The listing builds one solid part. Answer for the finished solid, in the listing's coordinates (mm). Face numbers are marked on the shaded views. A direction names the side the tool comes from. Coordinates: 2 decimals unless noted, no trailing zeros. Loops run counter-clockwise (first coordinate to the right, second up) from the corner with the lowest first, then second, coordinate; pieces in that order, holes last. Notation, with made-up numbers: (-3, 55) - (5, 55) arc R21 ccw to (5, 66) - close; hole circle Ø9 at (6, 81). An arc over 180 degrees is marked (long way). Put each result on its own line as item: value.
```python
from build123d import *

# Parameters (mm, degrees)
SKETCH1_W                       = 40
SKETCH1_H                       = 50
SKETCH1_R                       = 45
BOSS_EXTRUDE1_DEPTH             = 50
SKETCH3_R                       = 13
CUT_EXTRUDE1_DEPTH              = 130
BOSS_EXTRUDE3_DEPTH             = 42
BOSS_EXTRUDE3_DEPTH_BACK        = 10
SKETCH6_W                       = 7
SKETCH6_H                       = 4
SKETCH6_H_2                     = 10
SKETCH6_W_2                     = 3
CUT_EXTRUDE2_DEPTH              = 11
CUT_EXTRUDE2_DEPTH_BACK         = 43
SKETCH5_W                       = 42
SKETCH5_H                       = 40
SKETCH9_R                       = 1.5
CUT_EXTRUDE4_DEPTH              = 10
SKIZZE1_R                       = 6
SCHNITT_LINEAR_AUSTRAGEN1_DEPTH = 50
AUFSATZ_LINEAR_START            = 36
SKIZZE2_R                       = 17.5
SKIZZE2_R_2                     = 6
AUFSATZ_LINEAR_AUSTRAGEN1_DEPTH = 36
AUFSATZ_LINEAR_START_2          = 1
SKIZZE3_R                       = 21.5
SKIZZE3_R_2                     = 17.5
AUFSATZ_LINEAR_AUSTRAGEN2_DEPTH = 1
SKIZZE4_R                       = 1.65
SCHNITT_LINEAR_AUSTRAGEN2_DEPTH = 15
SKIZZE5_R                       = 18.5
SCHNITT_LINEAR_AUSTRAGEN3_DEPTH = 7
SKIZZE6_R                       = 17.25
SCHNITT_LINEAR_AUSTRAGEN4_DEPTH = 1


with BuildPart() as part:
    # Sketch1 → Boss-Extrude1 (new body)
    with BuildSketch(Plane.XY):
        with Locations((70, 60)):
            Rectangle(SKETCH1_W, SKETCH1_H)
        with BuildLine():
            Line((44.614473451, -5.877819215), (50, 35))
            Line((50, 35), (50, 85))
            Line((50, 85), (10, 85))
            Line((10, 85), (-35.25108577, 27.970715973))
            ThreePointArc((-35.25108577, 27.970715973), (14.810488519, 42.492933881), (45, 0))
            ThreePointArc((45, 0), (44.903514925, -2.945224501), (44.614473451, -5.877819215))
        make_face()
        Circle(SKETCH1_R)
    extrude(amount=BOSS_EXTRUDE1_DEPTH)

    # Sketch3 → Cut-Extrude1 (cut)
    with BuildSketch(Plane(origin=(90, 0, 0), x_dir=(0, 0, -1), z_dir=(1, 0, 0))):
        with Locations(Location((-25, 60, 0), (0, 0, 90))):
            Circle(SKETCH3_R)
    extrude(amount=-CUT_EXTRUDE1_DEPTH, mode=Mode.SUBTRACT)

    # Sketch6 → Boss-Extrude3 (add, two sides: drawn at the far end of the back side and taken through both)
    with BuildSketch(Plane(origin=(0, 85, 0), x_dir=(1, 0, 0), z_dir=(0, 1, 0)).offset(-BOSS_EXTRUDE3_DEPTH_BACK)):
        Polygon((43, -4), (43, 0), (10, 0), (10, -4), (13, -4), align=None)
        with Locations((6.5, -2)):
            Rectangle(SKETCH6_W, SKETCH6_H)
        with Locations((6.5, -9)):
            Rectangle(SKETCH6_W, SKETCH6_H_2)
        with Locations((11.5, -9)):
            Rectangle(SKETCH6_W_2, SKETCH6_H_2)
        with Locations((11.5, -41)):
            Rectangle(SKETCH6_W_2, SKETCH6_H_2)
        with Locations((6.5, -41)):
            Rectangle(SKETCH6_W, SKETCH6_H_2)
        with Locations((6.5, -48)):
            Rectangle(SKETCH6_W, SKETCH6_H)
        Polygon((13, -46), (10, -46), (10, -50), (43, -50), (43, -46), align=None)
    extrude(amount=BOSS_EXTRUDE3_DEPTH + BOSS_EXTRUDE3_DEPTH_BACK)

    # Sketch5 → Cut-Extrude2 (cut, two sides: drawn at the far end of the back side and taken through both)
    with BuildSketch(Plane.ZY.offset(40).offset(-CUT_EXTRUDE2_DEPTH_BACK)):
        with Locations((25, 60)):
            Rectangle(SKETCH5_W, SKETCH5_H)
    extrude(amount=CUT_EXTRUDE2_DEPTH + CUT_EXTRUDE2_DEPTH_BACK, mode=Mode.SUBTRACT)

    # Sketch9 → Cut-Extrude4 (cut)
    with BuildSketch(Plane(origin=(13, 0, 0), x_dir=(0, 0, -1), z_dir=(1, 0, 0))):
        with Locations(Location((-9.500219356, 121.499780644, 0), (0, 0, 90))):
            Circle(SKETCH9_R)
        with Locations(Location((-9.500219356, 90.500219356, 0), (0, 0, 90))):
            Circle(SKETCH9_R)
        with Locations(Location((-40.499780644, 90.500219356, 0), (0, 0, 90))):
            Circle(SKETCH9_R)
        with Locations(Location((-40.499780644, 121.499780644, 0), (0, 0, 90))):
            Circle(SKETCH9_R)
    extrude(amount=-CUT_EXTRUDE4_DEPTH, mode=Mode.SUBTRACT)

    # Skizze1 → Schnitt-Linear austragen1 (cut)
    with BuildSketch(Plane(origin=(0, 0, 0), x_dir=(-1, 0, 0), z_dir=(0, 0, -1))):
        Circle(SKIZZE1_R)
    extrude(amount=-SCHNITT_LINEAR_AUSTRAGEN1_DEPTH, mode=Mode.SUBTRACT)

    # Skizze2 → Aufsatz-Linear austragen1 (add)
    with BuildSketch(Plane(origin=(0, 0, 0), x_dir=(-1, 0, 0), z_dir=(0, 0, -1)).offset(AUFSATZ_LINEAR_START)):
        with Locations(Location((0, 0, 0), (0, 0, 180))):
            Circle(SKIZZE2_R)
        Circle(SKIZZE2_R_2, mode=Mode.SUBTRACT)
    extrude(amount=-AUFSATZ_LINEAR_AUSTRAGEN1_DEPTH)

    # Skizze3 → Aufsatz-Linear austragen2 (add)
    with BuildSketch(Plane(origin=(0, 0, 0), x_dir=(-1, 0, 0), z_dir=(0, 0, -1)).offset(AUFSATZ_LINEAR_START_2)):
        with Locations(Location((0, 0, 0), (0, 0, 180))):
            Circle(SKIZZE3_R)
        Circle(SKIZZE3_R_2, mode=Mode.SUBTRACT)
    extrude(amount=-AUFSATZ_LINEAR_AUSTRAGEN2_DEPTH)

    # Skizze4 → Schnitt-Linear austragen2 (cut)
    with BuildSketch(Plane(origin=(0, 0, -36), x_dir=(-1, 0, 0), z_dir=(0, 0, -1))):
        with Locations((-11.75, 0)):
            Circle(SKIZZE4_R)
        with Locations((-5.875, 10.175798494)):
            Circle(SKIZZE4_R)
        with Locations((5.875, 10.175798494)):
            Circle(SKIZZE4_R)
        with Locations((11.75, 0)):
            Circle(SKIZZE4_R)
        with Locations((5.875, -10.175798494)):
            Circle(SKIZZE4_R)
        with Locations((-5.875, -10.175798494)):
            Circle(SKIZZE4_R)
    extrude(amount=-SCHNITT_LINEAR_AUSTRAGEN2_DEPTH, mode=Mode.SUBTRACT)

    # Skizze5 → Schnitt-Linear austragen3 (cut)
    with BuildSketch(Plane(origin=(90, 0, 0), x_dir=(0, 0, -1), z_dir=(1, 0, 0))):
        with Locations(Location((-25, 60, 0), (0, 0, 90))):
            Circle(SKIZZE5_R)
    schnitt_linear_austragen3 = extrude(amount=-SCHNITT_LINEAR_AUSTRAGEN3_DEPTH, mode=Mode.SUBTRACT)

    # Skizze6 → Schnitt-Linear austragen4 (cut)
    with BuildSketch(Plane(origin=(83, 0, 0), x_dir=(0, 0, -1), z_dir=(1, 0, 0))):
        with Locations(Location((-25, 60, 0), (0, 0, 90))):
            Circle(SKIZZE6_R)
    schnitt_linear_austragen4 = extrude(amount=-SCHNITT_LINEAR_AUSTRAGEN4_DEPTH, mode=Mode.SUBTRACT)

    # Spiegeln1: Schnitt-Linear austragen3, Schnitt-Linear austragen4 across plane
    add(schnitt_linear_austragen3.mirror(Plane(origin=(46.5, 0, 0), x_dir=(0, 0, 1), z_dir=(1, 0, 0))), mode=Mode.SUBTRACT)
    add(schnitt_linear_austragen4.mirror(Plane(origin=(46.5, 0, 0), x_dir=(0, 0, 1), z_dir=(1, 0, 0))), mode=Mode.SUBTRACT)


solid = part.part
```
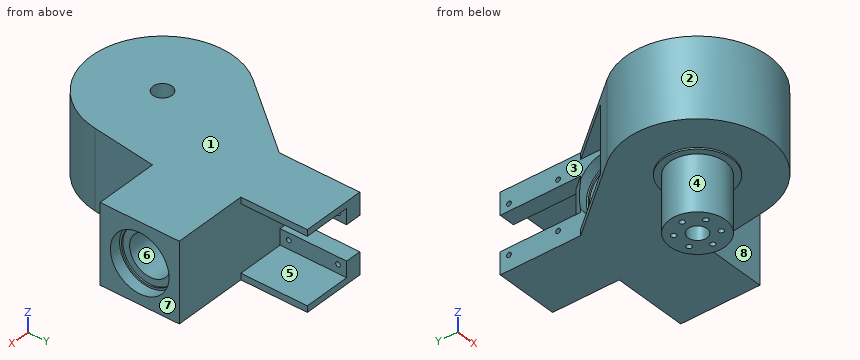
1) For the marked faces 4, 5, 6, 7 and 8, determine the directions among +Z, -Z, +X, -X, +Y, -Y from which every point of the face is accessible in a straight line to the end or side of a thin tool.
Found:
face 4: -Z
face 5: +X, +Y
face 6: +X, -X
face 7: +Z, -Z, +X, +Y, -Y
face 8: +Z, -Z, +X, -Y
2) The part is cut by section D-D (x = 38). Give the vertices of the cut face in (y, z).
Found:
outline: (-24.1, 0) - (127, 0) - (127, 4) - (85, 4) - (85, 46) - (127, 46) - (127, 50) - (-24.1, 50) - close; hole circle Ø26 at (60, 25)
3) Straight lines are drawn through the part: L1, parallel to Z at x = 39, y = 60; L2, parallel to Z at x = -29, y = 18; L3, parallel to X at y = 72, z = 6. For each, find the intervals that lie inside material, in ascending order. Write a range as [from, to].
Found:
L1: z = [0, 12], [38, 50]
L2: z = [0, 50]
L3: x = [3, 90]
4) Each of these flat-tipped pins is pushed along its axis until it touches: pin 1 (17 mm diameter, centred on y = 56.5, z = 29, fed in from +X); pin 2 (10.5 mm diameter, centred on y = 52.5, z = 33.5, fed in from -X); pin 3 (12 mm diameter, centred on x = 61, z = 25, fed in from -Y); pin 4 (1.5 mm diameter, centred on x = 3, y = -3.5, fed in from +Z). Where does it stop, or does it pass through?
Found:
pin 1: stops at x = 82
pin 2: stops at x = 11
pin 3: stops at y = 35
pin 4: passes through
5) The part is cut by section C-C (x = 0). Give the vertices of the cut face in (y, z).
Found:
outline: (-45, 0) - (-21.5, 0) - (-21.5, -1) - (-17.5, -1) - (-17.5, -36) - (-6, -36) - (-6, 50) - (-45, 50) - close; (6, -36) - (17.5, -36) - (17.5, -1) - (21.5, -1) - (21.5, 0) - (72.4, 0) - (72.4, 4) - (40, 4) - (40, 46) - (72.4, 46) - (72.4, 50) - (6, 50) - close
6) The part is cut by section B-B (z = 25). State how many separate pieces and enclosed holes the cut face has, and give its area (3 significant figures).
Found:
separate pieces: 2
enclosed holes: 1
area: 8,180 mm^2
7) The part is cut by section A-A (y = 111). Give the vertices of the cut face in (x, z), and give its area (3 significant figures).
Found:
outline: (3, 0) - (43, 0) - (43, 4) - (13, 4) - (13, 14) - (3, 14) - close; (3, 36) - (13, 36) - (13, 46) - (43, 46) - (43, 50) - (3, 50) - close
area: 520 mm^2
8) For a pull along Z with two mould halves and no side action, classify the marked faces 1, 2 and 3 as pulls with the +Z half, pulls with the -Z half, needs draft (parallel to the pull), parting line crosses it, or undercut.
Found:
face 1: pulls with the +Z half
face 2: needs draft
face 3: undercut
